```python
from build123d import *

# Parameters (mm, degrees)
EXTRUDE_1_DEPTH = 91
FILLET_1_SIZE   = 3
FILLET_1_SIZE_2 = 2
FILLET_2_SIZE   = 3
FILLET_2_SIZE_2 = 2


with BuildPart() as part:
    # ｽｹｯﾁ1 → ﾎﾞｽ - 押し出し1 (new body)
    with BuildSketch(Plane.XY):
        with BuildLine():
            Line((20, -11), (-20, -11))
            ThreePointArc((-20, -11), (-31, 0), (-20, 11))
            Line((-20, 11), (20, 11))
            ThreePointArc((20, 11), (31, 0), (20, -11))
        make_face()
    extrude(amount=EXTRUDE_1_DEPTH)

    # ﾌｨﾚｯﾄ1
    # an asymmetric fillet: 3, 2 mm, written as the material it takes off along each edge
    with BuildSketch(Plane(origin=(20, -11, 91), x_dir=(0, 0, -1), z_dir=(-1, 0, 0)), Plane(origin=(-20, 11, 91), x_dir=(0, 0, -1), z_dir=(1, 0, 0))) as fillet_1_piece_1:
        with BuildLine():
            Bezier((FILLET_1_SIZE, 0), (0, 0), (0, -FILLET_1_SIZE_2), weights=[1, 0.707106781, 1])
            Line((0, -FILLET_1_SIZE_2), (0, 0))
            Line((0, 0), (FILLET_1_SIZE, 0))
        make_face()
    extrude(amount=40, mode=Mode.SUBTRACT)
    with BuildSketch(Plane(origin=(20, 0, 91), x_dir=(0, 1, 0), z_dir=(-1, 0, 0))) as fillet_1_piece_2:
        with BuildLine():
            Bezier((11, FILLET_1_SIZE), (11, 0), (11 - FILLET_1_SIZE_2, 0), weights=[1, 0.707106781, 1])
            Line((11 - FILLET_1_SIZE_2, 0), (11, 0))
            Line((11, 0), (11, FILLET_1_SIZE))
        make_face()
    revolve(axis=Axis((20, 0, 91), (0, 0, -1)), revolution_arc=180, mode=Mode.SUBTRACT)
    with BuildSketch(Plane(origin=(-20, 0, 91), x_dir=(0, -1, 0), z_dir=(1, 0, 0))) as fillet_1_piece_3:
        with BuildLine():
            Bezier((11, FILLET_1_SIZE), (11, 0), (11 - FILLET_1_SIZE_2, 0), weights=[1, 0.707106781, 1])
            Line((11 - FILLET_1_SIZE_2, 0), (11, 0))
            Line((11, 0), (11, FILLET_1_SIZE))
        make_face()
    revolve(axis=Axis((-20, 0, 91), (0, 0, -1)), revolution_arc=180, mode=Mode.SUBTRACT)

    # ﾌｨﾚｯﾄ2
    # an asymmetric fillet: 3, 2 mm, written as the material it takes off along each edge
    with BuildSketch(Plane(origin=(20, -11, 0), x_dir=(0, 0, 1), z_dir=(-1, 0, 0))) as fillet_2_piece_1:
        with BuildLine():
            Bezier((FILLET_2_SIZE, 0), (0, 0), (0, FILLET_2_SIZE_2), weights=[1, 0.707106781, 1])
            Line((0, FILLET_2_SIZE_2), (0, 0))
            Line((0, 0), (FILLET_2_SIZE, 0))
        make_face()
    extrude(amount=40, mode=Mode.SUBTRACT)
    with BuildSketch(Plane(origin=(-20, 0, 0), x_dir=(0, -1, 0), z_dir=(1, 0, 0))) as fillet_2_piece_2:
        with BuildLine():
            Bezier((11 - FILLET_2_SIZE_2, 0), (11, 0), (11, -FILLET_2_SIZE), weights=[1, 0.707106781, 1])
            Line((11, -FILLET_2_SIZE), (11, 0))
            Line((11, 0), (11 - FILLET_2_SIZE_2, 0))
        make_face()
    revolve(axis=Axis((-20, 0, 0), (0, 0, -1)), revolution_arc=180, mode=Mode.SUBTRACT)
    with BuildSketch(Plane(origin=(-20, 11, 0), x_dir=(0, -1, 0), z_dir=(1, 0, 0))) as fillet_2_piece_3:
        with BuildLine():
            Bezier((FILLET_2_SIZE_2, 0), (0, 0), (0, -FILLET_2_SIZE), weights=[1, 0.707106781, 1])
            Line((0, -FILLET_2_SIZE), (0, 0))
            Line((0, 0), (FILLET_2_SIZE_2, 0))
        make_face()
    extrude(amount=40, mode=Mode.SUBTRACT)
    with BuildSketch(Plane(origin=(20, 0, 0), x_dir=(0, 1, 0), z_dir=(-1, 0, 0))) as fillet_2_piece_4:
        with BuildLine():
            Bezier((11 - FILLET_2_SIZE_2, 0), (11, 0), (11, -FILLET_2_SIZE), weights=[1, 0.707106781, 1])
            Line((11, -FILLET_2_SIZE), (11, 0))
            Line((11, 0), (11 - FILLET_2_SIZE_2, 0))
        make_face()
    revolve(axis=Axis((20, 0, 0), (0, 0, -1)), revolution_arc=180, mode=Mode.SUBTRACT)


solid = part.part
```
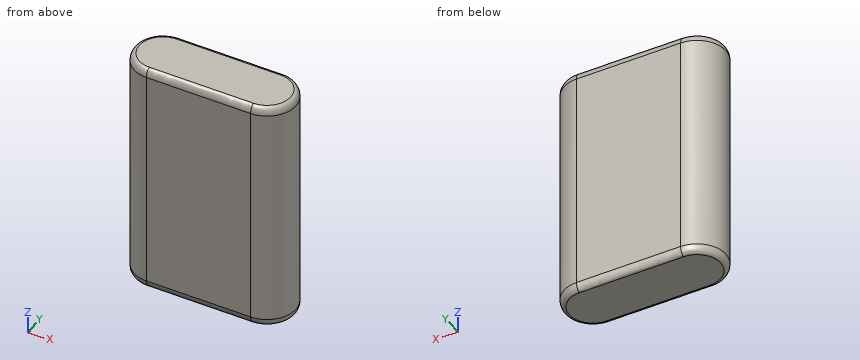
Build history of the part. All positions in model axes, mm. Round coordinates to 2 decimals unless told otherwise and drop trailing zeros. Loops run counter-clockwise (first coordinate to the right, second up) from the corner with the lowest first, then second, coordinate; pieces in that order, holes last.
Item 1: Pin check, flat tip, straight feed: P1, Ø5, axis at y = -4.5, z = 42.5, coming from the +X side. Stop position of the tip, or through.
Item 2: Saw through at A-A (z = 45). List the corners of the cut face in (x, y), then the cut area to 3 significant figures.
Item 3: Drill centre lines: line 1 along X through (y, z) = (-9, 60); line 2 along Y through (x, z) = (-23, 8); line 3 along X through (y, z) = (-4, 37). Where is each one in solid material? Low to high.
Worked answers:
1. P1: stops at x = 30.82
2. outline: (-20, -11) - (20, -11) arc R11 ccw to (20, 11) - (-20, 11) arc R11 ccw to start
2. area: 1,260 mm2
3. line 1: x = -26.32 to 26.32
3. line 2: y = -10.58 to 10.58
3. line 3: x = -30.25 to 30.25
